Can you work these out from the drawing? Everything is in mm from the part's minimum corner. Coordinates: 2 decimals unless noted, no trailing zeros. Order: outer loops, then holes, each group sorted by start corner. A loop starts at its lowest first (then second) coordinate and runs counter-clockwise, first axis right, second up. Notation, with made-up numbers: (55.5, 37.25) -> (81.5, 37.25) arc R20 ccw to (81.5, 49.25) -> close; hole circle Ø2 at (68, 83.25). An arc over 180 degrees is marked (long way). Answer in a Markdown table with one row per item.
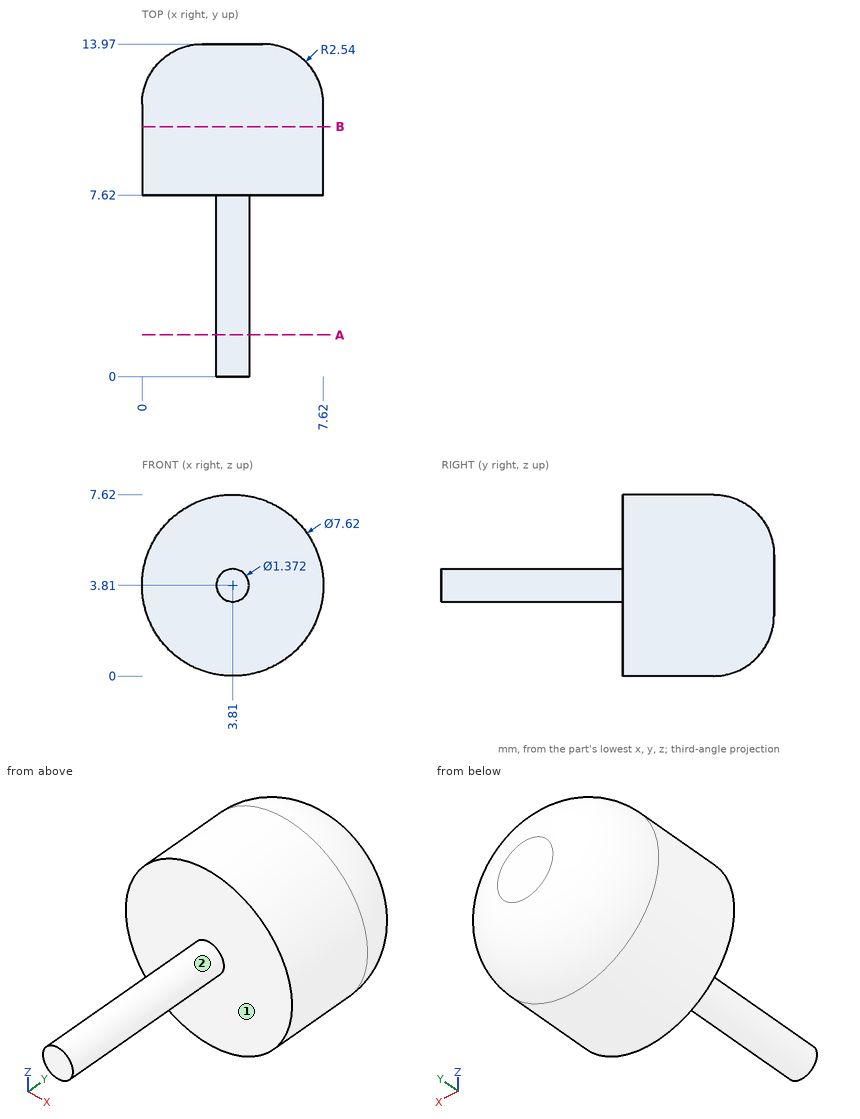
(1) Suppose I cut it at A-A (y = 1.75). Please give me the cut outline in (x, z) (1 decimal).
Response values:
| item | result |
|---|---|
| outline | circle Ø1.4 at (3.8, 3.8) |
(2) Suppose I cut it at B-B (y = 10.5). Please give me the cut outline in (x, z), and give its area (3 significant figures).
Response values:
| item | result |
|---|---|
| outline | circle Ø7.62 at (3.81, 3.81) |
| area | 45.6 mm2 |
(3) Will these pins go through, and if not, where does the flat tip stop? pin 1 Ø1 at (x, y) = (3.5, 1.5) entering from +Z; pin 2 Ø1.5 at (y, z) = (3.5, 4) entering from +X; pin 3 Ø1.5 at (x, z) = (3, 2.5) entering from -Y.
Response values:
| item | result |
|---|---|
| pin 1 | z = 4.5 |
| pin 2 | x = 4.5 |
| pin 3 | y = 7.62 |
(4) I need wall thicknesses on line 1 (Y direction, x = 4.25, z = 2.5); line 2 (Z direction, x = 3.5, y = 4.5); line 3 (Y direction, x = 1.5, z = 1.25) (1 decimal). Which ranges of each line are inside material? Lowest first, please. Write a range as [from, to].
Response values:
| item | result |
|---|---|
| line 1 | [7.62, 13.97] |
| line 2 | [3.2, 4.42] |
| line 3 | [7.6, 12.7] |
(5) We'd pull the mould along X, two halves only. Please class the marked faces 1 and 2: +X half, -X half, draft (parallel to the pull), parting line (faces both ways), or undercut.
Response values:
| item | result |
|---|---|
| face 1 | draft |
| face 2 | parting line |
